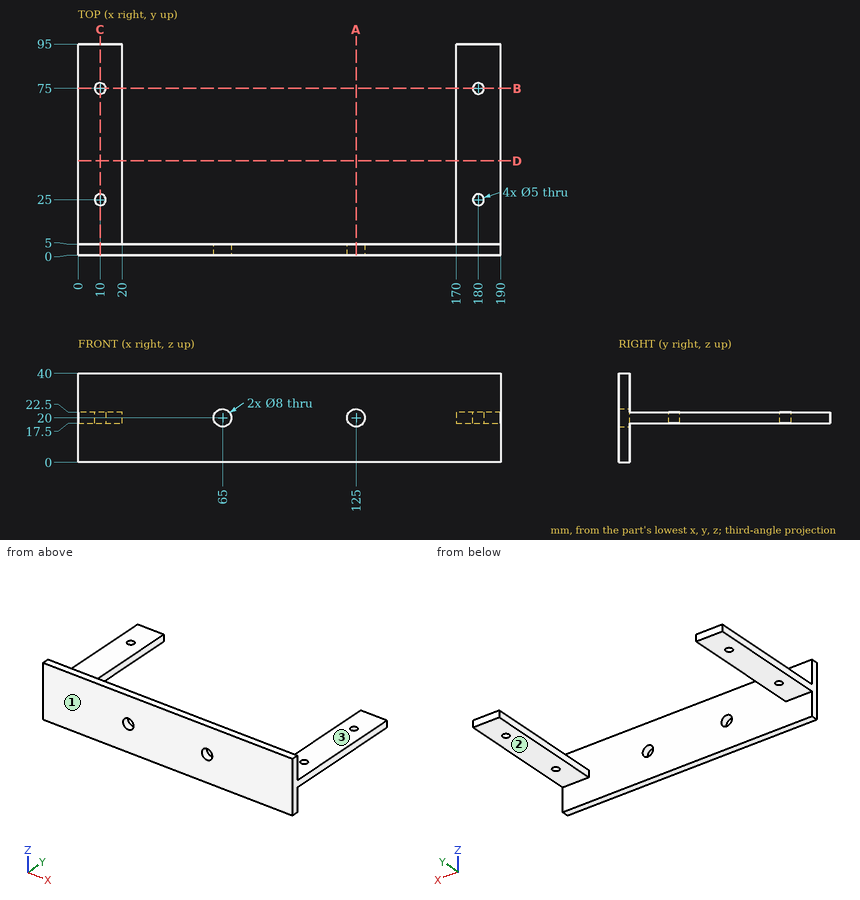
Drawing for the job (mm, zero at the part's lowest x, y, z). A direction names the side the tool comes from. Round coordinates to 2 decimals unless told otherwise and drop trailing zeros. Write each loop counter-clockwise with the first axis right and the second up, starting at its lowest first coordinate (ties: lowest second). Pieces come first, ordered by that corner, then holes.
Item 1: Band-saw the part on B-B on y = 75. Write the cut outline in (x, z), then the cut area to 3 significant figures.
Filled in:
outline: (0, 17.5) - (7.5, 17.5) - (7.5, 22.5) - (0, 22.5) - close; (12.5, 17.5) - (20, 17.5) - (20, 22.5) - (12.5, 22.5) - close; (170, 17.5) - (177.5, 17.5) - (177.5, 22.5) - (170, 22.5) - close; (182.5, 17.5) - (190, 17.5) - (190, 22.5) - (182.5, 22.5) - close
area: 150 mm2
Item 2: Band-saw the part on D-D on y = 42.5. Write the cut outline in (x, z), then the cut area to 3 significant figures.
Filled in:
outline: (0, 17.5) - (20, 17.5) - (20, 22.5) - (0, 22.5) - close; (170, 17.5) - (190, 17.5) - (190, 22.5) - (170, 22.5) - close
area: 200 mm2
Item 3: Band-saw the part on C-C on x = 10. Write the cut outline in (y, z).
Filled in:
outline: (0, 0) - (5, 0) - (5, 17.5) - (22.5, 17.5) - (22.5, 22.5) - (5, 22.5) - (5, 40) - (0, 40) - close; (27.5, 17.5) - (72.5, 17.5) - (72.5, 22.5) - (27.5, 22.5) - close; (77.5, 17.5) - (95, 17.5) - (95, 22.5) - (77.5, 22.5) - close
Item 4: Band-saw the part on A-A on x = 125. Write the cut outline in (y, z).
Filled in:
outline: (0, 0) - (5, 0) - (5, 16) - (0, 16) - close; (0, 24) - (5, 24) - (5, 40) - (0, 40) - close
Item 5: Drill centre lines: L1, parallel to X at y = 2, z = 20; L2, parallel to Y at x = 180, z = 21; L3, parallel to Y at x = 103.5, z = 4. Where is each one in solid material? Low to high.
Filled in:
L1: x = 0 to 61, 69 to 121, 129 to 190
L2: y = 0 to 22.5, 27.5 to 72.5, 77.5 to 95
L3: y = 0 to 5
Item 6: Drop flat-ended pins along their axis: pin 1 Ø2.5 at (y, z) = (62.5, 20) entering from -X; pin 2 Ø13 at (x, z) = (65, 20) entering from +Y; pin 3 Ø10 at (x, y) = (181.5, 68.5) entering from +Z; pin 4 Ø22 at (x, y) = (183, 41) entering from -Z. Give the stop position or say it passes through.
Filled in:
pin 1: stops at x = 0
pin 2: stops at y = 5
pin 3: stops at z = 22.5
pin 4: stops at z = 17.5
Item 7: Tool access for the marked faces 1, 2 and 3: list every direction of +Z, -Z, +X, -X, +Y, -Y with a clear straight run to the whole face (end or side of a thin tool).
Filled in:
face 1: +Z, -Z, +X, -X, -Y
face 2: -Z, +X, -X, +Y
face 3: +Z, +X, -X, +Y
